The listing builds one solid part. Answer for the finished solid, in the listing's coordinates (mm). A direction names the side the tool comes from. Give positions to 0.01 mm unless a question says otherwise; leave off trailing zeros. Write each loop counter-clockwise with the first axis right and the second up, starting at its lowest first coordinate (ties: lowest second). Pieces come first, ordered by that corner, then holes. Notation, with made-up numbers: (-3.75, 7) - (36.25, 7) arc R29 cw to (36.25, 38) - close; hole circle Ø5 at (68, 85.5). An arc over 180 degrees is marked (long way). Return JSON: item names as keys, results as strings.
from build123d import *

# Parameters (mm, degrees)
F0_W     = 600
F0_H     = 600
F1_DEPTH = 200
F2_R     = 180
F3_DEPTH = 200.001
F5_DEPTH = 200
F7_DEPTH = 150
F8_R     = 100
F9_DEPTH = 350.001


with BuildPart() as f1:
    # F0 (on Front) → F1 (new body)
    with BuildSketch(Plane.XZ):
        Rectangle(F0_W, F0_H)
    extrude(amount=F1_DEPTH)

    # F2 (on face) → F3 (cut, through all)
    with BuildSketch(Plane.XZ.offset(200)):
        with Locations((0, -300)):
            Circle(F2_R)
    extrude(amount=-F3_DEPTH, mode=Mode.SUBTRACT)

    # F4 (on face) → F5 (join)
    with BuildSketch(Plane.XZ.offset(200)):
        with BuildLine():
            Line((-300, 300), (300, 300))
            ThreePointArc((300, 300), (0, 600), (-300, 300))
        make_face()
    extrude(amount=-F5_DEPTH)

    # F6 (on face) → F7 (join)
    with BuildSketch(Plane.XZ.offset(200)):
        with BuildLine():
            Line((-180, 540), (-180, 60))
            ThreePointArc((-180, 60), (0, 0), (180, 60))
            Line((180, 60), (180, 540))
            ThreePointArc((180, 540), (0, 600), (-180, 540))
        make_face()
    extrude(amount=F7_DEPTH)

    # F8 (on face) → F9 (cut, through all)
    with BuildSketch(Plane.XZ.offset(350)):
        with Locations((0, 300)):
            Circle(F8_R)
    extrude(amount=-F9_DEPTH, mode=Mode.SUBTRACT)


solid = f1.part
Item 1: A cutting plane is placed at C-C on z = 174. Determine the outline of the cut face in (x, y).
Answer below:
{"outline": "(-300, -200) - (-180, -200) - (-180, -350) - (180, -350) - (180, -200) - (300, -200) - (300, 0) - (-300, 0) - close"}
Item 2: Flat-ended cylindrical pins translate along their axes: P1, Ø5, axis at y = -298.5, z = 62.5, coming from the -X side; P2, Ø1, axis at x = -123.5, y = -131, coming from the -Z side; P3, Ø1, axis at y = -140, z = 497.5, coming from the -X side. Find the tip coordinate at first contact, or state that the pin passes through.
Answer below:
{"P1": "stops at x = -180", "P2": "stops at z = -169.52", "P3": "stops at x = -226.25"}
Item 3: For faces 1 (the face through (-180, -274, 303)), 2 (the face through (-2.703, -273.95, 0.012)), 3 (the face through (180, -274, 297)), determine the directions among +Z, -Z, +X, -X, +Y, -Y from which every point of the face is accessible in a straight line to the end or side of a thin tool.
Answer below:
{"face 1": "+Z, -Z, -X, -Y", "face 2": "-Z, -Y", "face 3": "+Z, -Z, +X, -Y"}
Item 4: A cutting plane is placed at D-D on y = -122.5. Determine the outline of the cut face in (x, z).
Answer below:
{"outline": "(-300, -300) - (-180, -300) arc R180 cw to (180, -300) - (300, -300) - (300, 300) arc R300 ccw to (-300, 300) - close; hole circle Ø200 at (0, 300)"}
Item 5: Consider L1, parallel to Z at x = 0, y = -104; L2, parallel to Z at x = 0, y = -219; L3, parallel to Y at x = 131, z = -134.5. Determine where each line is inside the solid, lowest interval first.
Answer below:
{"L1": "z = -120 to 200, 400 to 600", "L2": "z = 0 to 200, 400 to 600", "L3": "y = -200 to 0"}
Item 6: A cutting plane is placed at A-A on x = 0. Determine the outline of the cut face in (y, z), then the cut area to 3 significant figures.
Answer below:
{"outline": "(-350, 0) - (-200, 0) - (-200, -120) - (0, -120) - (0, 200) - (-350, 200) - close; (-350, 400) - (0, 400) - (0, 600) - (-350, 600) - close", "area": "164,000 mm²"}
Item 7: The mould has two halves that part along X. Classify faces 4 (the face through (3.958, -101.4, -120.044)), 5 (the face through (300, -99, -4)), 6 (the face through (-21.68, -177.45, 202.38)), 7 (the face through (-4, -200, -61)): +X half, -X half, draft (parallel to the pull), parting line (faces both ways), or undercut.
Answer below:
{"face 4": "undercut", "face 5": "+X half", "face 6": "undercut", "face 7": "draft"}
Item 8: A cutting plane is placed at B-B on y = -244. Determine the outline of the cut face in (x, z), then the cut area to 3 significant figures.
Answer below:
{"outline": "(-180, 60) arc R300 ccw to (180, 60) - (180, 540) arc R300 ccw to (-180, 540) - close; hole circle Ø200 at (0, 300)", "area": "171,000 mm²"}
